The figure shows three views and two pictorial views of one solid part (mm, origin at its lowest corner). Answer the questions. Round coordinates to 2 decimals unless told otherwise and drop trailing zeros. Loops run counter-clockwise (first coordinate to the right, second up) from the corner with the lowest first, then second, coordinate; pieces in that order, holes last. Notation, with made-up numbers: (80, 13) -> (121, 13) arc R23 ccw to (121, 36) -> close; hole circle Ø4 at (75, -0.5). An arc over 180 degrees is marked (long way). Put each result on its own line as item: value.
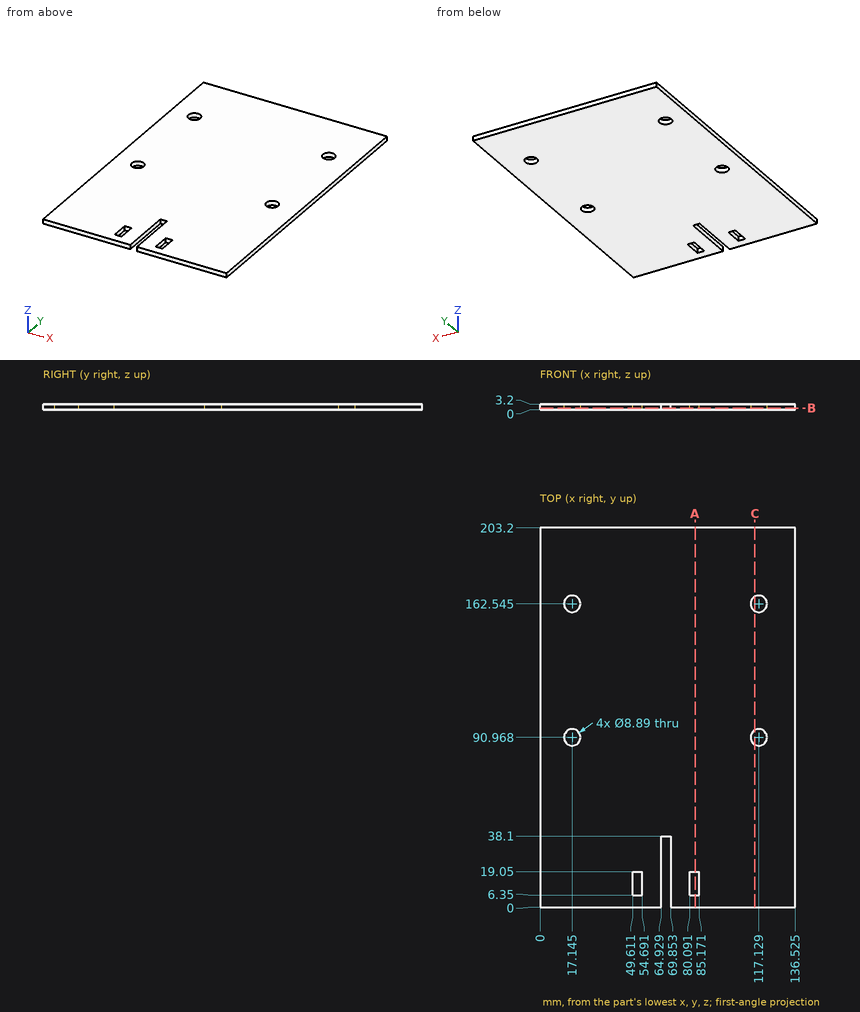
Item 1: A flat-ended cylindrical pin translates along its axis: pin 1 Ø1.6 at (x, z) = (66.5, 2) entering from -Y. Find the tip coordinate at first contact, or state that the pin passes through.
Derived:
pin 1: stops at y = 38.1
Item 2: The part is cut by section C-C (x = 115). Determine the outline of the cut face in (y, z).
Derived:
outline: (0, 0) -> (87.07, 0) -> (87.07, 3.2) -> (0, 3.2) -> close; (94.87, 0) -> (158.64, 0) -> (158.64, 3.2) -> (94.87, 3.2) -> close; (166.45, 0) -> (203.2, 0) -> (203.2, 3.2) -> (166.45, 3.2) -> close
Item 3: Find the intervals of material crossed by line 1 along X through (y, z) = (15, 2.05) (1 decimal); line 2 along X through (y, z) = (30, 1.9) (1 decimal), in increasing order.
Derived:
line 1: x = 0 to 49.6, 54.7 to 64.9, 69.9 to 80.1, 85.2 to 136.5
line 2: x = 0 to 64.9, 69.9 to 136.5
Item 4: The part is cut by section A-A (x = 83). Determine the outline of the cut face in (y, z).
Derived:
outline: (0, 0) -> (6.35, 0) -> (6.35, 3.2) -> (0, 3.2) -> close; (19.05, 0) -> (203.2, 0) -> (203.2, 3.2) -> (19.05, 3.2) -> close
Item 5: The part is cut by section B-B (z = 1). State how many separate pieces and enclosed holes the cut face has, then the cut area to 3 significant figures.
Derived:
separate pieces: 1
enclosed holes: 6
area: 27,200 mm^2
